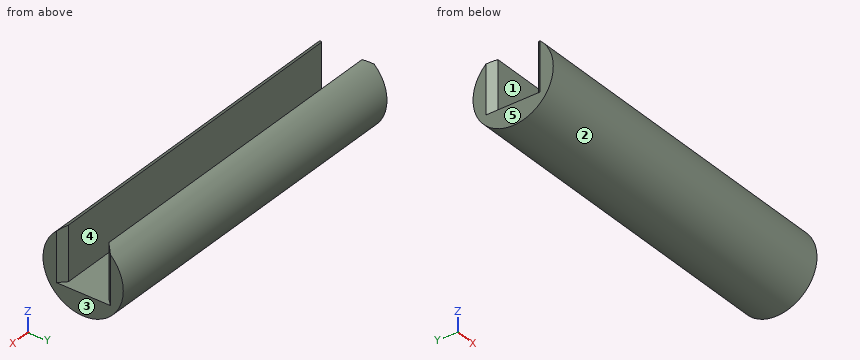
Solid Edge part; units mm, degrees
sketch "Sketch1" plane through (0, 0, 0) normal (1, 0, 0) x (0, 1, 0)
  circle A0 centre (0, 0) radius 17.5
extrude "Protrusion1" add sketch "Sketch1" along normal blind 150
sketch "Sketch2" plane through (150, 0, 0) normal (1, 0, 0) x (0, 1, 0)
  line L0 (8.9, -8.32) -> (8.9, 21.68)
  line L1 (8.9, 21.68) -> (-8.7, 21.68)
  line L2 (-8.7, 21.68) -> (-8.7, -8.32)
  line L3 (-8.7, -8.32) -> (8.9, -8.32)
extrude "ExtrudedCutout_1" cut sketch "Sketch2" against normal blind 150
chamfer "Chamfer_1" distance 3 angle 45 4 edges at (150, 8.9, 3.3739) (150, -8.7, 3.4321) (0, 8.9, 3.3739) (0, -8.7, 3.4321)
Source: CAD feature listing. Evaluate the final solid. Frame: model axes, mm. Face numbers are marked on the shaded views. A direction names the side the tool comes from. Coordinates: 2 decimals unless noted, no trailing zeros. Write each loop counter-clockwise with the first axis right and the second up, starting at its lowest first coordinate (ties: lowest second). Pieces come first, ordered by that corner, then holes. Notation, with made-up numbers: (48, -31.5) - (66, -31.5) arc R20 ccw to (66, -18.5) - close; hole circle Ø5 at (68, -1). An arc over 180 degrees is marked (long way). Answer as a JSON object with one key per item and string values.
Q1. Section query C-C, the plane y = 0. Output: boundary loops of the cut face in (x, z).
Ans:
{"outline": "(0, -17.5) - (150, -17.5) - (150, -8.32) - (0, -8.32) - close"}
Q2. Section query B-B, the plane x = 39. Output: boundary loops of the cut face in (y, z), plus the area to 3 significant figures.
Ans:
{"outline": "(-8.7, -8.32) - (-8.7, 15.18) arc R17.5 ccw (long way) to (8.9, 15.07) - (8.9, -8.32) - close", "area": "521 mm2"}
Q3. Section query A-A, the plane z = 0. Output: boundary loops of the cut face in (x, y).
Ans:
{"outline": "(0, -17.5) - (150, -17.5) - (150, -11.7) - (147, -8.7) - (3, -8.7) - (0, -11.7) - close; (0, 11.9) - (3, 8.9) - (147, 8.9) - (150, 11.9) - (150, 17.5) - (0, 17.5) - close"}
Q4. Section query D-D, the plane z = 6.5. Output: boundary loops of the cut face in (x, y), plus the area to 3 significant figures.
Ans:
{"outline": "(0, -16.25) - (150, -16.25) - (150, -11.7) - (147, -8.7) - (3, -8.7) - (0, -11.7) - close; (0, 11.9) - (3, 8.9) - (147, 8.9) - (150, 11.9) - (150, 16.25) - (0, 16.25) - close", "area": "2,220 mm2"}
Q5. Set-up query: the marked faces 4 and 5. Return all of +Z, -Z, +X, -X, +Y, -Y with unobstructed straight access to the full face (end or side cutting, diameter ignored); none if empty.
Ans:
{"face 4": "+Z, +X, -X", "face 5": "+Z, -Z, -X, +Y, -Y"}
Q6. First-contact query: pin 1 Ø6 at (x, z) = (87, -7) entering from +Y; pin 2 Ø10 at (x, y) = (92.5, -6.5) entering from +Z; pin 3 Ø10 at (x, y) = (69.5, -10) entering from -Z; pin 4 Ø12 at (x, y) = (116.5, -1.5) entering from -Z. Flat tips, straight axial feed; report the tip coordinate or a pass-through.
Ans:
{"pin 1": "stops at y = 17.04", "pin 2": "stops at z = 15.18", "pin 3": "stops at z = -16.77", "pin 4": "stops at z = -17.5"}
Q7. Draft query along Y for the marked faces 1, 2 and 3. Return one class per face: released by +Y, released by -Y, zero draft, split by the parting line, or undercut.
Ans:
{"face 1": "undercut", "face 2": "split by the parting line", "face 3": "zero draft"}
Q8. Material intervals for line 1 (Y direction, x = 70.5, z = -1); line 2 (Y direction, x = 115, z = 10); line 3 (Z direction, x = 7, y = -0.5), sorted ascending. Write a range as [from, to].
Ans:
{"line 1": "y = [-17.47, -8.7], [8.9, 17.47]", "line 2": "y = [-14.36, -8.7], [8.9, 14.36]", "line 3": "z = [-17.49, -8.32]"}
